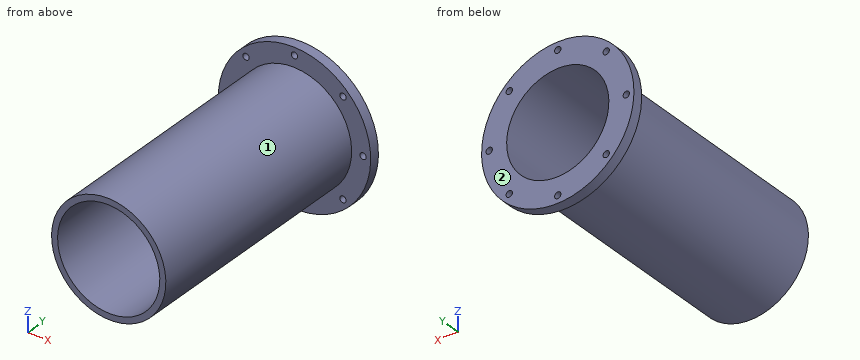
```python
from build123d import *

# Parameters (mm, degrees)
BOLT_HOLES_PROFILE_R = 3.175
BOLT_HOLES_DEPTH     = 276.914624476


with BuildPart() as part:
    # Shell Profile → Shell Revolve (revolve)
    with BuildSketch(Plane.XY, mode=Mode.PRIVATE) as shell_revolve_sk:
        Polygon((51.1302, 0), (51.1302, 254), (76.2, 254), (76.2, 243.84), (57.15, 243.84), (57.15, 0), align=None)
    revolve(shell_revolve_sk.sketch.rotate(Axis((0, 0, 0), (0, -1, 0)), 90), axis=Axis((0, 0, 0), (0, -1, 0)))

    # Bolt Holes Profile → Bolt Holes (cut, through all)
    with BuildSketch(Plane(origin=(0, 254, 0), x_dir=(1, 0, 0), z_dir=(0, 1, 0))):
        with Locations(Location((0, 68.58, 0), (0, 0, 270))):
            Circle(BOLT_HOLES_PROFILE_R)
        with Locations(Location((48.493383054, 48.493383054, 0), (0, 0, 270))):
            Circle(BOLT_HOLES_PROFILE_R)
        with Locations(Location((68.58, 0, 0), (0, 0, 270))):
            Circle(BOLT_HOLES_PROFILE_R)
        with Locations(Location((48.493383054, -48.493383054, 0), (0, 0, 270))):
            Circle(BOLT_HOLES_PROFILE_R)
        with Locations(Location((0, -68.58, 0), (0, 0, 270))):
            Circle(BOLT_HOLES_PROFILE_R)
        with Locations(Location((-48.493383054, -48.493383054, 0), (0, 0, 270))):
            Circle(BOLT_HOLES_PROFILE_R)
        with Locations(Location((-68.58, 0, 0), (0, 0, 270))):
            Circle(BOLT_HOLES_PROFILE_R)
        with Locations(Location((-48.493383054, 48.493383054, 0), (0, 0, 270))):
            Circle(BOLT_HOLES_PROFILE_R)
    extrude(amount=-BOLT_HOLES_DEPTH, mode=Mode.SUBTRACT)


solid = part.part
```
Geometry: final body of the model. Coordinates: model frame, mm. Face numbers are marked on the shaded views. A direction names the side the tool comes from. Coordinates: 2 decimals unless noted, no trailing zeros. Write each loop counter-clockwise with the first axis right and the second up, starting at its lowest first coordinate (ties: lowest second). Pieces come first, ordered by that corner, then holes. Notation, with made-up numbers: M -38,10 L 17,10 A16 cw 17,24 Z; hole C -11,34 d10. An arc over 180 degrees is marked long. Answer as CSV lines item,"result". Start each with the question number.
Q1. Line query: line 1 (Z direction, x = 2, y = 19) (3 decimals); line 2 (X direction, y = 87.5, z = -1.5); line 3 (Y direction, x = -52.5, z = 48). Output: solid intervals per line, ascending. Write a range as from..to.
Q2. Cut plane D-D on x = 68.58. Return the cut outline in (y, z) (3 decimals), then the cut area to 3 significant figures.
Q3. Reachability of the marked faces 1 and 2 from +Z, -Z, +X, -X, +Y, -Y: full face, straight path, thin tool, end or side. Return the list, or none.
Q4. Pin query (flat end, axial travel): P1, Ø7.5, axis at x = -48.49, z = 48.49, coming from the +Y side; P2, Ø10, axis at x = 68.58, z = 0, coming from the -Y side; P3, Ø5.5, axis at x = 48.49, z = -48.49, coming from the +Y side; P4, Ø4, axis at y = 188.5, z = 0.5, coming from the -X side. Return the tip coordinate at first contact, or that it passes through.
Q5. Cut plane C-C on z = -68.58. Return the cut outline in (x, y) (3 decimals).
Q6. Cut plane A-A on z = 0. Return the cut outline in (x, y) (3 decimals).
Q7. Cut plane B-B on x = 0. Return the cut outline in (y, z) (3 decimals), then the cut area to 3 significant figures.
Findings below:
1,line 1,"z = -57.115..-51.091, 51.091..57.115"
1,line 2,"x = -57.13..-51.11, 51.11..57.13"
1,line 3,"y = 243.84..254"
2,outline,"M 243.84,-33.215 L 254,-33.215 L 254,-3.175 L 243.84,-3.175 Z; M 243.84,3.175 L 254,3.175 L 254,33.215 L 243.84,33.215 Z"
2,area,"610 mm2"
3,face 1,"-Y"
3,face 2,"+Z, -Z, +X, -X, +Y"
4,P1,"stops at y = 254"
4,P2,"stops at y = 243.84"
4,P3,"passes through"
4,P4,"stops at x = -57.15"
5,outline,"M -33.215,243.84 L -3.175,243.84 L -3.175,254 L -33.215,254 Z; M 3.175,243.84 L 33.215,243.84 L 33.215,254 L 3.175,254 Z"
6,outline,"M -76.2,243.84 L -71.755,243.84 L -71.755,254 L -76.2,254 Z; M -65.405,243.84 L -57.15,243.84 L -57.15,0 L -51.13,0 L -51.13,254 L -65.405,254 Z; M 51.13,0 L 57.15,0 L 57.15,243.84 L 65.405,243.84 L 65.405,254 L 51.13,254 Z; M 71.755,243.84 L 76.2,243.84 L 76.2,254 L 71.755,254 Z"
7,outline,"M 0,-57.15 L 243.84,-57.15 L 243.84,-65.405 L 254,-65.405 L 254,-51.13 L 0,-51.13 Z; M 0,51.13 L 254,51.13 L 254,65.405 L 243.84,65.405 L 243.84,57.15 L 0,57.15 Z; M 243.84,-76.2 L 254,-76.2 L 254,-71.755 L 243.84,-71.755 Z; M 243.84,71.755 L 254,71.755 L 254,76.2 L 243.84,76.2 Z"
7,area,"3,320 mm2"
